Geometry check sheet. Reference: the model listing, model coordinates, mm. Face numbers are marked on the shaded views. A direction names the side the tool comes from. Give positions to 0.01 mm unless a question says otherwise; leave off trailing zeros. Loops run counter-clockwise (first coordinate to the right, second up) from the corner with the lowest first, then second, coordinate; pieces in that order, holes last. Notation, with made-up numbers: (-12, 29) -> (13, 29) arc R24 ccw to (13, 39) -> close; hole circle Ø5 at (43.25, 25.25). An arc over 180 degrees is marked (long way). Answer in a Markdown table with one row per item. Add a question column.
```python
from build123d import *

# Parameters (mm, degrees)
BOX003_W     = 50
BOX003_H     = 3.7
BOX003_DEPTH = 6
FILLET003_R  = 1.8
BOX_W        = 50
BOX_H        = 20
BOX_DEPTH    = 50
FILLET_R     = 1
BOX002_W     = 30
BOX002_H     = 30
BOX002_DEPTH = 4
FILLET002_R  = 2
BOX001_W     = 15
BOX001_H     = 26
BOX001_DEPTH = 23
FILLET001_R  = 2


with BuildPart() as fillet003:
    # Box003 → Box003 (new body)
    with BuildSketch(Plane(origin=(-20, -1.85, 15), x_dir=(1, 0, 0), z_dir=(0, 0, 1))):
        with Locations((25, 1.85)):
            Rectangle(BOX003_W, BOX003_H)
    extrude(amount=BOX003_DEPTH)

    # Fillet003
    fillet003_edges = [fillet003.edges().sort_by_distance(p)[0] for p in [
        (5, -1.85, 15),
        (5, -1.85, 21),
        (5, 1.85, 15),
        (5, 1.85, 21),
    ]]
    fillet(fillet003_edges, radius=FILLET003_R)


with BuildPart() as fusion001:
    # Box → Box (new body)
    with BuildSketch(Plane(origin=(0, -10, 0), x_dir=(1, 0, 0), z_dir=(0, 0, 1))):
        with Locations((25, 10)):
            Rectangle(BOX_W, BOX_H)
    extrude(amount=BOX_DEPTH)

    # Fillet
    fillet_edges = [fusion001.edges().sort_by_distance(p)[0] for p in [
        (0, -10, 25),
        (0, 10, 25),
    ]]
    fillet(fillet_edges, radius=FILLET_R)

    # Fusion001: union Fillet003
    add(fillet003.part)


with BuildPart() as fillet002:
    # Box002 → Box002 (new body)
    with BuildSketch(Plane(origin=(-10, -15, 0), x_dir=(1, 0, 0), z_dir=(0, 0, 1))):
        with Locations((15, 15)):
            Rectangle(BOX002_W, BOX002_H)
    extrude(amount=BOX002_DEPTH)

    # Fillet002
    fillet002_edges = [fillet002.edges().sort_by_distance(p)[0] for p in [
        (-10, -15, 2),
        (-10, 15, 2),
        (20, -15, 2),
        (20, 15, 2),
    ]]
    fillet(fillet002_edges, radius=FILLET002_R)


with BuildPart() as flood_sensor:
    # Box001 → Box001 (new body)
    with BuildSketch(Plane(origin=(-3, -13, 0), x_dir=(1, 0, 0), z_dir=(0, 0, 1))):
        with Locations((7.5, 13)):
            Rectangle(BOX001_W, BOX001_H)
    extrude(amount=BOX001_DEPTH)

    # Fillet001
    fillet001_edges = [flood_sensor.edges().sort_by_distance(p)[0] for p in [
        (-3, -13, 11.5),
        (-3, 13, 11.5),
        (12, 0, 23),
    ]]
    fillet(fillet001_edges, radius=FILLET001_R)

    # Fusion: union Fillet002
    add(fillet002.part)

    # Cut: cut Fusion001
    add(fusion001.part, mode=Mode.SUBTRACT)


solid = flood_sensor.part
```
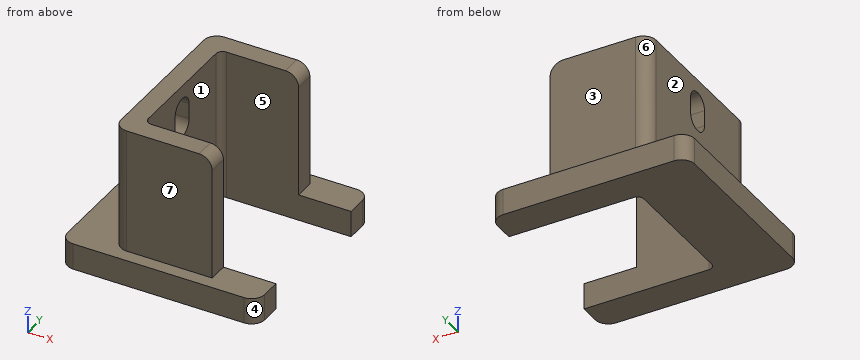
1. Sectioned sample at B-B (z = 18.25). Enter the section's corners in (x, y), plus the area to 3 significant figures.
2. Material ranges on L1, parallel to Y at x = 8.25, z = 7; L2, parallel to Z at x = 15, y = 11; L3, parallel to X at y = -10.75, z = 8.75, recorded low to high. Write a range as from..to.
3. Sectioned sample at C-C (y = 5.25). Enter the section's corners in (x, z).
4. Sectioned sample at D-D (x = -1.5). Enter the section's corners in (y, z).
5. Sectioned sample at A-A (x = 17). Enter the section's corners in (y, z).
6. Access from +Z, -Z, +X, -X, +Y, -Y to the whole of each face (thin tool, end or side, straight path). Record for the marked faces 5, 6 and 7.
7. Release check for a two-part mould opening along Y. For the marked faces 1, 2, 3 and 4 record: released by +Y, released by -Y, zero draft, split by the parting line, or undercut.
8. Gauge pin test, flat ends, axial feed: pin 1 Ø5 at (x, y) = (14, 11) entering from +Z; pin 2 Ø12 at (y, z) = (-6, 15.5) entering from +X; pin 3 Ø10.5 at (x, z) = (4, 11.5) entering from +Y. Record the tip position at first contact, or that the pin passes through.
Response:
| question | item | result |
|---|---|---|
| 1 | outline | (-3, -11) arc R2 ccw to (-1, -13) -> (12, -13) -> (12, -10) -> (1, -10) arc R1 cw to (0, -9) -> (0, -1.85) -> (-3, -1.85) -> close; (-3, 1.85) -> (0, 1.85) -> (0, 9) arc R1 cw to (1, 10) -> (12, 10) -> (12, 13) -> (-1, 13) arc R2 ccw to (-3, 11) -> close |
| 1 | area | 138 mm2 |
| 2 | L1 | y = -13..-10, 10..13 |
| 2 | L2 | z = 0..4 |
| 2 | L3 | x = -3..12 |
| 3 | outline | (-10, 0) -> (0, 0) -> (0, 23) -> (-3, 23) -> (-3, 4) -> (-10, 4) -> close |
| 4 | outline | (-15, 0) -> (15, 0) -> (15, 4) -> (12.94, 4) -> (12.94, 23) -> (-12.94, 23) -> (-12.94, 4) -> (-15, 4) -> close; hole (-1.85, 16.8) arc R1.8 ccw to (-0.05, 15) -> (0.05, 15) arc R1.8 ccw to (1.85, 16.8) -> (1.85, 19.2) arc R1.8 ccw to (0.05, 21) -> (-0.05, 21) arc R1.8 ccw to (-1.85, 19.2) -> close |
| 5 | outline | (-15, 0) -> (-10, 0) -> (-10, 4) -> (-15, 4) -> close; (10, 0) -> (15, 0) -> (15, 4) -> (10, 4) -> close |
| 6 | face 5 | +Z, -Z, +X |
| 6 | face 6 | +Z, -X, +Y |
| 6 | face 7 | +Z, +X, -X, -Y |
| 7 | face 1 | undercut |
| 7 | face 2 | zero draft |
| 7 | face 3 | released by +Y |
| 7 | face 4 | released by -Y |
| 8 | pin 1 | stops at z = 22.32 |
| 8 | pin 2 | stops at x = 12 |
| 8 | pin 3 | stops at y = 13 |
